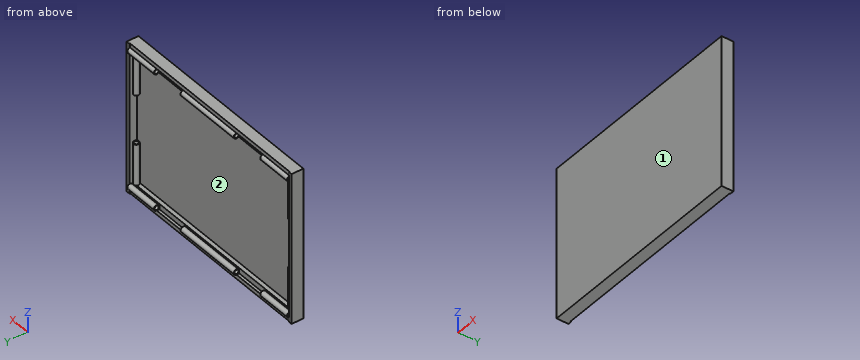
from build123d import *

# Parameters (mm, degrees)
SKETCH_1_W                 = 310
SKETCH_1_H                 = 220
EXTRUDE_1_DEPTH            = 12
SKETCH_8_W                 = 310
SKETCH_8_H                 = 10
EXTRUDE_12_DEPTH           = 4
SKETCH_10_R                = 4
CUT_EXTRUDE_5_DEPTH        = 305
SKETCH_11_W                = 4
SKETCH_11_H                = 4
EXTRUDE_13_DEPTH           = 5
EXTRUDE_START              = 300
SKETCH_12_R                = 4
SKETCH_12_R_2              = 3
EXTRUDE_1_2_DEPTH          = 300
SKETCH_15_W                = 5
SKETCH_15_H                = 220
EXTRUDE_15_DEPTH           = 5
SPLIT_START                = -99.339622642
SPLIT_BODIES_1_OUTLINE_R   = 3
SPLIT_BODIES_1_DEPTH       = 50
SPLIT_START_2              = 50.660377358
SPLIT_BODIES_1_2_OUTLINE_R = 3
SPLIT_BODIES_1_2_DEPTH     = 50
SKETCH_16_W                = 50
SKETCH_16_H                = 8
EXTRUDE_16_DEPTH           = 12
SKETCH_19_W                = 300
SKETCH_19_H                = 192.127016654
CUT_EXTRUDE_6_DEPTH        = 6
SKETCH_22_W                = 4
SKETCH_22_H                = 192.127016654
EXTRUDE_17_DEPTH           = 4
SKETCH_23_R                = 4
CUT_EXTRUDE_8_DEPTH        = 192.127016654
SKETCH_23_3_R              = 4
SKETCH_23_3_R_2            = 3
EXTRUDE_2_DEPTH            = 192.127016654
SPLIT_START_3              = -58.830188679
SPLIT_BODIES_2_OUTLINE_R   = 3
SPLIT_BODIES_2_DEPTH       = 72
SPLIT_START_4              = -58.957205333
SPLIT_BODIES_2_2_OUTLINE_R = 3
SPLIT_BODIES_2_2_DEPTH     = 0.127016654
SKETCH_24_W                = 8
SKETCH_24_H                = 72
SKETCH_24_H_2              = 72.127016654
EXTRUDE_18_DEPTH           = 6


# Read off the part's stored shape, not the designer's step: 分割1, 分割2
with BuildPart() as part:
    # 草图1 → Extrude 1 (new body)
    with BuildSketch(Plane(origin=(0, 0, 0), x_dir=(1, 0, 0), z_dir=(0, 1, 0))):
        with Locations((0.660377358, 22.830188679)):
            Rectangle(SKETCH_1_W, SKETCH_1_H)
    extrude(amount=EXTRUDE_1_DEPTH)

    # 草图8 → 凸台-拉伸12 (add)
    with BuildSketch(Plane(origin=(0, 12, 0), x_dir=(1, 0, 0), z_dir=(0, 1, 0))):
        with Locations((0.660377358, 127.830188679)):
            Rectangle(SKETCH_8_W, SKETCH_8_H)
        with Locations((0.660377358, -82.169811321)):
            Rectangle(SKETCH_8_W, SKETCH_8_H)
    extrude(amount=EXTRUDE_12_DEPTH)

    # 草图10 → 切除-拉伸5 (cut)
    with BuildSketch(Plane(origin=(155.660377358, 0, 0), x_dir=(0, 0, -1), z_dir=(1, 0, 0))):
        with Locations((-77.169811321, 16)):
            Circle(SKETCH_10_R)
        with Locations((122.830188679, 16)):
            Circle(SKETCH_10_R)
    extrude(amount=-CUT_EXTRUDE_5_DEPTH, mode=Mode.SUBTRACT)

    # 草图11 → 凸台-拉伸13 (add)
    with BuildSketch(Plane(origin=(155.660377358, 0, 0), x_dir=(0, 0, -1), z_dir=(1, 0, 0))):
        with Locations((-79.169811321, 14)):
            Rectangle(SKETCH_11_W, SKETCH_11_H)
        with Locations((124.830188679, 14)):
            Rectangle(SKETCH_11_W, SKETCH_11_H)
    extrude(amount=-EXTRUDE_13_DEPTH)

    # 草图12 → Extrude 1 2 (add)
    # profile 1 of 2: a face of its own
    with BuildSketch(Plane(origin=(-149.339622642, 0, 0), x_dir=(0, 0, -1), z_dir=(1, 0, 0)).offset(EXTRUDE_START)):
        with Locations((-77.169811321, 16)):
            Circle(SKETCH_12_R)
        with Locations((-77.169811321, 16)):
            Circle(SKETCH_12_R_2, mode=Mode.SUBTRACT)
    # profile 2 of 2: a face of its own
    with BuildSketch(Plane(origin=(-149.339622642, 0, 0), x_dir=(0, 0, -1), z_dir=(1, 0, 0)).offset(EXTRUDE_START)):
        with Locations((122.830188679, 16)):
            Circle(SKETCH_12_R)
        with Locations((122.830188679, 16)):
            Circle(SKETCH_12_R_2, mode=Mode.SUBTRACT)
    extrude(amount=-EXTRUDE_1_2_DEPTH)

    # 草图15 → 凸台-拉伸15 (add)
    with BuildSketch(Plane(origin=(0, 12, 0), x_dir=(1, 0, 0), z_dir=(0, 1, 0))):
        with Locations((-151.839622642, 22.830188679)):
            Rectangle(SKETCH_15_W, SKETCH_15_H)
        with Locations((153.160377358, 22.830188679)):
            Rectangle(SKETCH_15_W, SKETCH_15_H)
    extrude(amount=EXTRUDE_15_DEPTH)

    # Split Bodies 1 outline → Split Bodies 1 (cut)
    # profile 1 of 2: a face of its own
    with BuildSketch(Plane.YZ.offset(SPLIT_START)):
        with BuildLine():
            ThreePointArc((12, 77.169811321), (18.828427125, 74.341384196), (16, 81.169811321))
            Line((16, 81.169811321), (0, 81.169811321))
            Line((0, 81.169811321), (0, 73.169811321))
            Line((0, 73.169811321), (12, 73.169811321))
            Line((12, 73.169811321), (12, 77.169811321))
        make_face()
        with Locations((16, 77.169811321)):
            Circle(SPLIT_BODIES_1_OUTLINE_R, mode=Mode.SUBTRACT)
    # profile 2 of 2: a face of its own
    with BuildSketch(Plane.YZ.offset(SPLIT_START)):
        with BuildLine():
            Line((12, -118.830188679), (0, -118.830188679))
            Line((0, -118.830188679), (0, -126.830188679))
            Line((0, -126.830188679), (16, -126.830188679))
            ThreePointArc((16, -126.830188679), (18.828427125, -120.001761554), (12, -122.830188679))
            Line((12, -122.830188679), (12, -118.830188679))
        make_face()
        with Locations((16, -122.830188679)):
            Circle(SPLIT_BODIES_1_OUTLINE_R, mode=Mode.SUBTRACT)
    extrude(amount=SPLIT_BODIES_1_DEPTH, mode=Mode.SUBTRACT)

    # Split Bodies 1 2 outline → Split Bodies 1 2 (cut)
    # profile 1 of 2: a face of its own
    with BuildSketch(Plane.YZ.offset(SPLIT_START_2)):
        with BuildLine():
            ThreePointArc((12, 77.169811321), (18.828427125, 74.341384196), (16, 81.169811321))
            Line((16, 81.169811321), (0, 81.169811321))
            Line((0, 81.169811321), (0, 73.169811321))
            Line((0, 73.169811321), (12, 73.169811321))
            Line((12, 73.169811321), (12, 77.169811321))
        make_face()
        with Locations((16, 77.169811321)):
            Circle(SPLIT_BODIES_1_2_OUTLINE_R, mode=Mode.SUBTRACT)
    # profile 2 of 2: a face of its own
    with BuildSketch(Plane.YZ.offset(SPLIT_START_2)):
        with BuildLine():
            Line((12, -118.830188679), (0, -118.830188679))
            Line((0, -118.830188679), (0, -126.830188679))
            Line((0, -126.830188679), (16, -126.830188679))
            ThreePointArc((16, -126.830188679), (18.828427125, -120.001761554), (12, -122.830188679))
            Line((12, -122.830188679), (12, -118.830188679))
        make_face()
        with Locations((16, -122.830188679)):
            Circle(SPLIT_BODIES_1_2_OUTLINE_R, mode=Mode.SUBTRACT)
    extrude(amount=SPLIT_BODIES_1_2_DEPTH, mode=Mode.SUBTRACT)

    # 草图16 → 凸台-拉伸16 (add)
    with BuildSketch(Plane(origin=(0, 12, 0), x_dir=(1, 0, 0), z_dir=(0, 1, 0))):
        with Locations((-74.339622642, 122.830188679)):
            Rectangle(SKETCH_16_W, SKETCH_16_H)
        with Locations((75.660377358, 122.830188679)):
            Rectangle(SKETCH_16_W, SKETCH_16_H)
        with Locations((-74.339622642, -77.169811321)):
            Rectangle(SKETCH_16_W, SKETCH_16_H)
        with Locations((75.660377358, -77.169811321)):
            Rectangle(SKETCH_16_W, SKETCH_16_H)
    extrude(amount=-EXTRUDE_16_DEPTH)

    # 草图19 → 切除-拉伸6 (cut)
    with BuildSketch(Plane(origin=(0, 12, 0), x_dir=(1, 0, 0), z_dir=(0, 1, 0))):
        with Locations((0.660377358, 22.893697006)):
            Rectangle(SKETCH_19_W, SKETCH_19_H)
    extrude(amount=-CUT_EXTRUDE_6_DEPTH, mode=Mode.SUBTRACT)

    # 草图22 → 凸台-拉伸17 (add)
    with BuildSketch(Plane(origin=(0, 6, 0), x_dir=(1, 0, 0), z_dir=(0, 1, 0))):
        with Locations((-147.339622642, 22.893697006)):
            Rectangle(SKETCH_22_W, SKETCH_22_H)
        with Locations((148.660377358, 22.893697006)):
            Rectangle(SKETCH_22_W, SKETCH_22_H)
    extrude(amount=EXTRUDE_17_DEPTH)

    # 草图23 → 切除-拉伸8 (cut)
    with BuildSketch(Plane.XY.offset(-118.957205333)):
        with Locations((-145.339622642, 10)):
            Circle(SKETCH_23_R)
        with Locations((146.660377358, 10)):
            Circle(SKETCH_23_R)
    extrude(amount=CUT_EXTRUDE_8_DEPTH, mode=Mode.SUBTRACT)

    # 草图23<3> → 拉伸-薄壁2 (add)
    # profile 1 of 2: a face of its own
    with BuildSketch(Plane.XY.offset(-118.957205333)):
        with Locations((-145.339622642, 10)):
            Circle(SKETCH_23_3_R)
        with Locations((-145.339622642, 10)):
            Circle(SKETCH_23_3_R_2, mode=Mode.SUBTRACT)
    # profile 2 of 2: a face of its own
    with BuildSketch(Plane.XY.offset(-118.957205333)):
        with Locations((146.660377358, 10)):
            Circle(SKETCH_23_3_R)
        with Locations((146.660377358, 10)):
            Circle(SKETCH_23_3_R_2, mode=Mode.SUBTRACT)
    extrude(amount=EXTRUDE_2_DEPTH)

    # Split Bodies 2 outline → Split Bodies 2 (cut)
    # profile 1 of 2: a face of its own
    with BuildSketch(Plane.XY.offset(SPLIT_START_3)):
        with BuildLine():
            Line((-149.339622642, 0), (-141.339622642, 0))
            Line((-141.339622642, 0), (-141.339622642, 6))
            Line((-141.339622642, 6), (-145.339622642, 6))
            ThreePointArc((-145.339622642, 6), (-142.511195517, 12.828427125), (-149.339622642, 10))
            Line((-149.339622642, 10), (-149.339622642, 0))
        make_face()
        with Locations((-145.339622642, 10)):
            Circle(SPLIT_BODIES_2_OUTLINE_R, mode=Mode.SUBTRACT)
    # profile 2 of 2: a face of its own
    with BuildSketch(Plane.XY.offset(SPLIT_START_3)):
        with BuildLine():
            Line((142.660377358, 6), (142.660377358, 0))
            Line((142.660377358, 0), (150.660377358, 0))
            Line((150.660377358, 0), (150.660377358, 10))
            ThreePointArc((150.660377358, 10), (143.831950234, 12.828427125), (146.660377358, 6))
            Line((146.660377358, 6), (142.660377358, 6))
        make_face()
        with Locations((146.660377358, 10)):
            Circle(SPLIT_BODIES_2_OUTLINE_R, mode=Mode.SUBTRACT)
    extrude(amount=SPLIT_BODIES_2_DEPTH, mode=Mode.SUBTRACT)

    # Split Bodies 2 2 outline → Split Bodies 2 2 (cut)
    with BuildSketch(Plane.XY.offset(SPLIT_START_4)):
        with BuildLine():
            Line((142.660377358, 6), (142.660377358, 0))
            Line((142.660377358, 0), (150.660377358, 0))
            Line((150.660377358, 0), (150.660377358, 10))
            ThreePointArc((150.660377358, 10), (143.831950234, 12.828427125), (146.660377358, 6))
            Line((146.660377358, 6), (142.660377358, 6))
        make_face()
        with Locations((146.660377358, 10)):
            Circle(SPLIT_BODIES_2_2_OUTLINE_R, mode=Mode.SUBTRACT)
    extrude(amount=SPLIT_BODIES_2_2_DEPTH, mode=Mode.SUBTRACT)

    # 草图24 → 凸台-拉伸18 (add)
    with BuildSketch(Plane(origin=(0, 6, 0), x_dir=(1, 0, 0), z_dir=(0, 1, 0))):
        with Locations((-145.339622642, 22.830188679)):
            Rectangle(SKETCH_24_W, SKETCH_24_H)
        with Locations((146.660377358, 22.893697006)):
            Rectangle(SKETCH_24_W, SKETCH_24_H_2)
    extrude(amount=-EXTRUDE_18_DEPTH)


solid = part.part
Verification items for the finished model (mm, model axes). Face numbers are marked on the shaded views. Coordinates: 2 decimals unless noted, no trailing zeros. Order: outer loops, then holes, each group sorted by start corner. A loop starts at its lowest first (then second) coordinate and runs counter-clockwise, first axis right, second up. Notation, with made-up numbers: M 13.25,5.25 L 68.25,5.25 A19 ccw 68.25,35.25 Z; hole C -39,-14 d2. An arc over 180 degrees is marked long. Return JSON: item names as keys, results as strings.
1) Thickness scan on L1, parallel to Z at x = -51, y = 14.25; L2, parallel to X at y = 14.5, z = 15; L3, parallel to Z at x = 29, y = 10.5. Record the ranges inside material, lowest first. Write a range as [from, to].
Answer list:
{"L1": "[-132.83, -126.83], [81.17, 87.17]", "L2": "[-154.34, -149.34], [150.66, 155.66]", "L3": "[-132.83, -118.96], [73.17, 87.17]"}
2) Cross-section at A-A, the plane x = 24. Record the boundary of the cut face in (y, z), and give its area (3 significant figures).
Answer list:
{"outline": "M 0,-132.83 L 16,-132.83 L 16,-126.83 A4 ccw long 12,-122.83 L 12,-118.96 L 6,-118.96 L 6,73.17 L 12,73.17 L 12,77.17 A4 ccw long 16,81.17 L 16,87.17 L 0,87.17 Z; hole C 16,-122.83 d6; hole C 16,77.17 d6", "area": "1,590 mm2"}
3) Cross-section at C-C, the plane x = 77.5. Record the boundary of the cut face in (y, z), and give its area (3 significant figures).
Answer list:
{"outline": "M 0,-132.83 L 16,-132.83 L 16,-126.83 L 12,-126.83 L 12,-118.96 L 6,-118.96 L 6,73.17 L 12,73.17 L 12,81.17 L 16,81.17 L 16,87.17 L 0,87.17 Z", "area": "1,540 mm2"}
4) Release check for a two-part mould opening along Z. For the marked faces 1 and 2 record: +Z half, -Z half, draft (parallel to the pull), parting line (faces both ways), or undercut.
Answer list:
{"face 1": "draft", "face 2": "undercut"}
5) Gauge pin test, flat ends, axial feed: pin 1 (4 mm diameter, centred on x = 71.5, z = -85, fed in from +Y); pin 2 (5.5 mm diameter, centred on x = 154.5, z = -75, fed in from +Y); pin 3 (2 mm diameter, centred on x = 70, z = 13, fed in from -Y). Record the tip position at first contact, or that the pin passes through.
Answer list:
{"pin 1": "y = 6", "pin 2": "y = 17", "pin 3": "y = 0"}
6) Cross-section at B-B, the plane z = -27.5. Record the boundary of the cut face in (x, y), and give its area (3 significant figures).
Answer list:
{"outline": "M -154.34,0 L 155.66,0 L 155.66,17 L 150.66,17 L 150.66,6 L -149.34,6 L -149.34,17 L -154.34,17 Z", "area": "1,970 mm2"}
